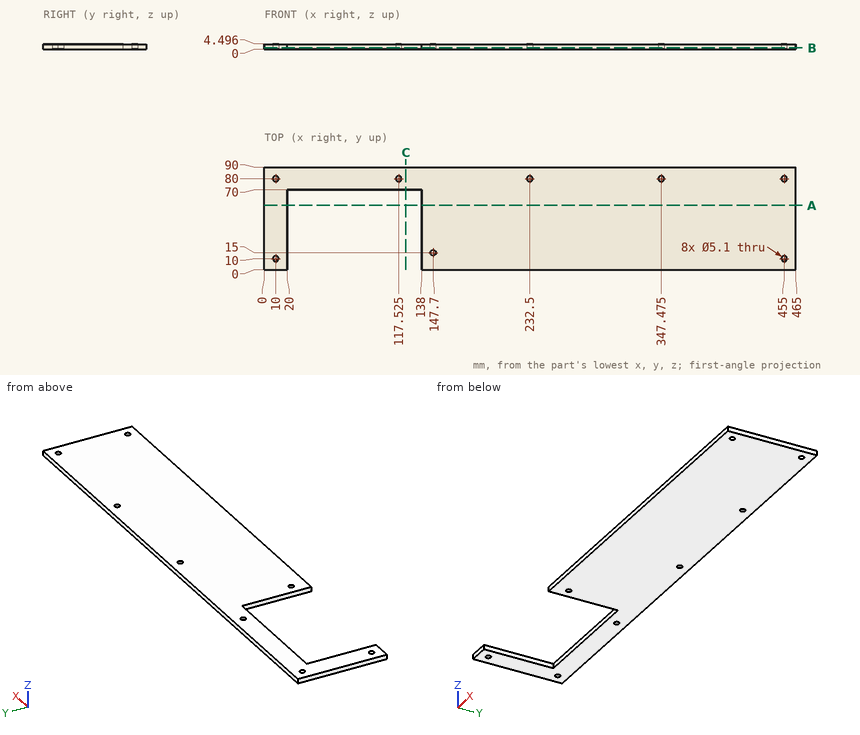
Design review of the part shown in the three views and the two pictorial views. Dimensions are in mm from the part's minimum x, y and z. Round coordinates to 2 decimals unless told otherwise and drop trailing zeros. Loops run counter-clockwise (first coordinate to the right, second up) from the corner with the lowest first, then second, coordinate; pieces in that order, holes last.
Q1. Insertion check: pin 1 Ø3 at (x, y) = (455, 10) entering from -Z. The pin has a flat end and moves straight along its axis. Give the tip position at first contact, or say it passes through.
Result sheet:
pin 1: passes through
Q2. Add section B-B on z = 1.1. Give the number of separate pieces and of enclosed holes in the cut face, plus the area to 3 significant figures.
Result sheet:
separate pieces: 1
enclosed holes: 8
area: 33,400 mm2
Q3. Add section A-A on y = 56.5. Write out the cut boundary in (x, z), plus the area to 3 significant figures.
Result sheet:
outline: (0, 0) - (20, 0) - (20, 4.5) - (0, 4.5) - close; (138, 0) - (465, 0) - (465, 4.5) - (138, 4.5) - close
area: 1,560 mm2
Q4. Add section C-C on x = 124. Write out the cut boundary in (y, z), plus the area to 3 significant figures.
Result sheet:
outline: (70, 0) - (90, 0) - (90, 4.5) - (70, 4.5) - close
area: 89.9 mm2
Q5. To check wall thickness, follow line 1 along Y through (x, z) = (455, 3.2); line 2 along Y through (x, z) = (147.7, 2.85); line 3 along Y through (x, z) = (232.5, 2). State the ranges of each line that lie inside material, in increasing order.
Result sheet:
line 1: y = 0 to 7.45, 12.55 to 77.45, 82.55 to 90
line 2: y = 0 to 12.45, 17.55 to 90
line 3: y = 0 to 77.45, 82.55 to 90
